Geometry: final body of the model. Coordinates: model frame, mm. Face numbers are marked on the shaded views. A direction names the side the tool comes from. Give positions to 0.01 mm unless a question says otherwise; leave off trailing zeros. Order: outer loops, then holes, each group sorted by start corner. A loop starts at its lowest first (then second) coordinate and runs counter-clockwise, first axis right, second up. Notation, with made-up numbers: (18, -20) -> (39, -20) arc R37 cw to (39, 18) -> close; hole circle Ø11 at (0, 83). An arc over 180 degrees is marked (long way). Answer in a Markdown table with one row per item. Add a question column.
Q1. Pull-direction query (Y, two-part tool) for the marked faces 3, 4 and 5; classes: +Y half, -Y half, draft (parallel to the pull), parting line (faces both ways), or undercut.
Q2. Cut plane C-C on y = -24. Return the cut outline in (x, z).
Q3. Cut plane D-D on z = 2. Return the cut outline in (x, y).
Q4. Line query: line 1 along Y through (x, z) = (0, 10.8); line 2 along X through (y, z) = (0, 10.8); line 3 along Z through (x, y) = (-5, -25). Output: solid intervals per line, ascending. Write a range as from..to.
Q5. Cut plane A-A on x = 0. Return the cut outline in (y, z).
Q6. Set-up query: the marked faces 1 and 2. Return all of +Z, -Z, +X, -X, +Y, -Y with unobstructed straight access to the full face (end or side cutting, diameter ignored); none if empty.
Q7. Contact query for flat-ended pins moving along their axis: P1, Ø1.5, axis at y = -21, z = 7.5, coming from the +X side; P2, Ø2.5, axis at y = -6, z = 7, coming from the -X side; P3, Ø2, axis at y = -19, z = 5, coming from the -X side. Output: stop coordinate, or through.
Q8. Cut plane B-B on z = 8. Return the cut outline in (x, y).
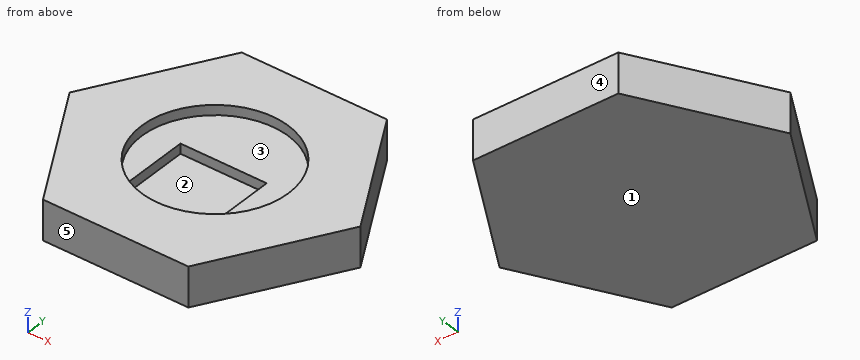
from build123d import *

# Parameters (mm, degrees)
PAD_DEPTH    = 9
SKETCH001_W  = 26.1
SKETCH001_H  = 34.4
POCKET_DEPTH = 3
SKETCH002_R  = 22.22
PAD001_DEPTH = 3


with BuildPart() as part:
    # Sketch → Pad (new body)
    with BuildSketch(Plane.XY):
        Polygon((44, 0), (22, 38.105118), (-22, 38.105118), (-44, 0), (-22, -38.105118), (22, -38.105118), align=None)
    extrude(amount=PAD_DEPTH)

    # Sketch001 (on Face8 of Pad) → Pocket (cut)
    with BuildSketch(Plane.XY.offset(9)):
        with Locations((0, -13.905118)):
            Rectangle(SKETCH001_W, SKETCH001_H)
    extrude(amount=-POCKET_DEPTH, mode=Mode.SUBTRACT)

    # Sketch002 (on Face5 of Pocket) → Pad001 (join)
    with BuildSketch(Plane.XY.offset(9)):
        Polygon((22, 38.105118), (-22, 38.105118), (-44, 0), (-22, -38.105118), (22, -38.105118), (44, 0), align=None)
        Circle(SKETCH002_R, mode=Mode.SUBTRACT)
    extrude(amount=PAD001_DEPTH)


solid = part.part
Completed:
| question | item | result |
|---|---|---|
| 1 | face 3 | undercut |
| 1 | face 4 | +Y half |
| 1 | face 5 | -Y half |
| 2 | outline | (-30.14, 0) -> (30.14, 0) -> (30.14, 12) -> (-30.14, 12) -> close; hole (-13.05, 6) -> (13.05, 6) -> (13.05, 9) -> (-13.05, 9) -> close |
| 3 | outline | (-44, 0) -> (-22, -38.11) -> (22, -38.11) -> (44, 0) -> (22, 38.11) -> (-22, 38.11) -> close |
| 4 | line 1 | y = -38.11..-22.22, 22.22..38.11 |
| 4 | line 2 | x = -44..-22.22, 22.22..44 |
| 4 | line 3 | z = 0..6, 9..12 |
| 5 | outline | (-38.11, 0) -> (38.11, 0) -> (38.11, 12) -> (22.22, 12) -> (22.22, 9) -> (3.29, 9) -> (3.29, 6) -> (-31.11, 6) -> (-31.11, 9) -> (-22.22, 9) -> (-22.22, 12) -> (-38.11, 12) -> close |
| 6 | face 1 | -Z, +X, -X, +Y, -Y |
| 6 | face 2 | none |
| 7 | P1 | stops at x = 32.31 |
| 7 | P2 | stops at x = -41.26 |
| 7 | P3 | stops at x = -33.61 |
| 8 | outline | (-44, 0) -> (-22, -38.11) -> (22, -38.11) -> (44, 0) -> (22, 38.11) -> (-22, 38.11) -> close; hole (-13.05, -31.11) -> (13.05, -31.11) -> (13.05, 3.29) -> (-13.05, 3.29) -> close |
